The listing builds one solid part. Answer for the finished solid, in the listing's coordinates (mm). Face numbers are marked on the shaded views. Round coordinates to 2 decimals unless told otherwise and drop trailing zeros. Order: outer loops, then holes, each group sorted by start corner. A loop starts at its lowest first (then second) coordinate and runs counter-clockwise, first axis right, second up. Notation, with made-up numbers: (67.5, 60.5) -> (84.5, 60.5) arc R28 cw to (84.5, 79.5) -> close; hole circle Ø7 at (43.25, 60). An arc over 180 degrees is marked (long way). Answer in a Markdown table with one row per item. Add a question column.
```python
from build123d import *

# Parameters (mm, degrees)
F1_DEPTH = 1.2
F2_DEPTH = 10
F3_DEPTH = 7
F4_SIZE2 = 8
F4_SIZE  = 1.4


with BuildPart() as f1:
    # F0 (on Top) → F1 (new body)
    with BuildSketch(Plane.XY):
        with BuildLine():
            Line((81.8, 59.8), (-81.8, 59.8))
            ThreePointArc((-81.8, 59.8), (-83.9213203436, 58.9213203436), (-84.8, 56.8))
            Line((-84.8, 56.8), (-84.8, -56.8))
            ThreePointArc((-84.8, -56.8), (-83.9213203436, -58.9213203436), (-81.8, -59.8))
            Line((-81.8, -59.8), (81.8, -59.8))
            ThreePointArc((81.8, -59.8), (83.9213203436, -58.9213203436), (84.8, -56.8))
            Line((84.8, -56.8), (84.8, 56.8))
            ThreePointArc((84.8, 56.8), (83.9213203436, 58.9213203436), (81.8, 59.8))
        make_face()
        with BuildLine():
            ThreePointArc((83.2, -55.2), (82.3213203436, -57.3213203436), (80.2, -58.2))
            Line((80.2, -58.2), (-80.2, -58.2))
            ThreePointArc((-80.2, -58.2), (-82.3213203436, -57.3213203436), (-83.2, -55.2))
            Line((-83.2, -55.2), (-83.2, 55.2))
            ThreePointArc((-83.2, 55.2), (-82.3213203436, 57.3213203436), (-80.2, 58.2))
            Line((-80.2, 58.2), (80.2, 58.2))
            ThreePointArc((80.2, 58.2), (82.3213203436, 57.3213203436), (83.2, 55.2))
            Line((83.2, 55.2), (83.2, -55.2))
        make_face(mode=Mode.SUBTRACT)
        with BuildLine():
            Line((-80.2, -58.2), (80.2, -58.2))
            ThreePointArc((80.2, -58.2), (82.3213203436, -57.3213203436), (83.2, -55.2))
            Line((83.2, -55.2), (83.2, 55.2))
            ThreePointArc((83.2, 55.2), (82.3213203436, 57.3213203436), (80.2, 58.2))
            Line((80.2, 58.2), (-80.2, 58.2))
            ThreePointArc((-80.2, 58.2), (-82.3213203436, 57.3213203436), (-83.2, 55.2))
            Line((-83.2, 55.2), (-83.2, -55.2))
            ThreePointArc((-83.2, -55.2), (-82.3213203436, -57.3213203436), (-80.2, -58.2))
        make_face()
        with BuildLine():
            ThreePointArc((-81.2, 53.2), (-80.3213203436, 55.3213203436), (-78.2, 56.2))
            Line((-78.2, 56.2), (78.2, 56.2))
            ThreePointArc((78.2, 56.2), (80.3213203436, 55.3213203436), (81.2, 53.2))
            Line((81.2, 53.2), (81.2, -53.2))
            ThreePointArc((81.2, -53.2), (80.3213203436, -55.3213203436), (78.2, -56.2))
            Line((78.2, -56.2), (-78.2, -56.2))
            ThreePointArc((-78.2, -56.2), (-80.3213203436, -55.3213203436), (-81.2, -53.2))
            Line((-81.2, -53.2), (-81.2, 53.2))
        make_face(mode=Mode.SUBTRACT)
        with BuildLine():
            Line((78.2, 56.2), (-78.2, 56.2))
            ThreePointArc((-78.2, 56.2), (-80.3213203436, 55.3213203436), (-81.2, 53.2))
            Line((-81.2, 53.2), (-81.2, -53.2))
            ThreePointArc((-81.2, -53.2), (-80.3213203436, -55.3213203436), (-78.2, -56.2))
            Line((-78.2, -56.2), (78.2, -56.2))
            ThreePointArc((78.2, -56.2), (80.3213203436, -55.3213203436), (81.2, -53.2))
            Line((81.2, -53.2), (81.2, 53.2))
            ThreePointArc((81.2, 53.2), (80.3213203436, 55.3213203436), (78.2, 56.2))
        make_face()
        with BuildLine():
            ThreePointArc((-80, 52), (-79.1213203436, 54.1213203436), (-77, 55))
            Line((-77, 55), (77, 55))
            ThreePointArc((77, 55), (79.1213203436, 54.1213203436), (80, 52))
            Line((80, 52), (80, -52))
            ThreePointArc((80, -52), (79.1213203436, -54.1213203436), (77, -55))
            Line((77, -55), (-77, -55))
            ThreePointArc((-77, -55), (-79.1213203436, -54.1213203436), (-80, -52))
            Line((-80, -52), (-80, 52))
        make_face(mode=Mode.SUBTRACT)
        with BuildLine():
            Line((77, 55), (-77, 55))
            ThreePointArc((-77, 55), (-79.1213203436, 54.1213203436), (-80, 52))
            Line((-80, 52), (-80, -52))
            ThreePointArc((-80, -52), (-79.1213203436, -54.1213203436), (-77, -55))
            Line((-77, -55), (77, -55))
            ThreePointArc((77, -55), (79.1213203436, -54.1213203436), (80, -52))
            Line((80, -52), (80, 52))
            ThreePointArc((80, 52), (79.1213203436, 54.1213203436), (77, 55))
        make_face()
    extrude(amount=F1_DEPTH)

    # F0 (on Top) → F2 (join)
    with BuildSketch(Plane.XY):
        with BuildLine():
            Line((78.2, 56.2), (-78.2, 56.2))
            ThreePointArc((-78.2, 56.2), (-80.3213203436, 55.3213203436), (-81.2, 53.2))
            Line((-81.2, 53.2), (-81.2, -53.2))
            ThreePointArc((-81.2, -53.2), (-80.3213203436, -55.3213203436), (-78.2, -56.2))
            Line((-78.2, -56.2), (78.2, -56.2))
            ThreePointArc((78.2, -56.2), (80.3213203436, -55.3213203436), (81.2, -53.2))
            Line((81.2, -53.2), (81.2, 53.2))
            ThreePointArc((81.2, 53.2), (80.3213203436, 55.3213203436), (78.2, 56.2))
        make_face()
        with BuildLine():
            ThreePointArc((-80, 52), (-79.1213203436, 54.1213203436), (-77, 55))
            Line((-77, 55), (77, 55))
            ThreePointArc((77, 55), (79.1213203436, 54.1213203436), (80, 52))
            Line((80, 52), (80, -52))
            ThreePointArc((80, -52), (79.1213203436, -54.1213203436), (77, -55))
            Line((77, -55), (-77, -55))
            ThreePointArc((-77, -55), (-79.1213203436, -54.1213203436), (-80, -52))
            Line((-80, -52), (-80, 52))
        make_face(mode=Mode.SUBTRACT)
    extrude(amount=F2_DEPTH)

    # F0 (on Top) → F3 (join)
    with BuildSketch(Plane.XY):
        with BuildLine():
            Line((81.8, 59.8), (-81.8, 59.8))
            ThreePointArc((-81.8, 59.8), (-83.9213203436, 58.9213203436), (-84.8, 56.8))
            Line((-84.8, 56.8), (-84.8, -56.8))
            ThreePointArc((-84.8, -56.8), (-83.9213203436, -58.9213203436), (-81.8, -59.8))
            Line((-81.8, -59.8), (81.8, -59.8))
            ThreePointArc((81.8, -59.8), (83.9213203436, -58.9213203436), (84.8, -56.8))
            Line((84.8, -56.8), (84.8, 56.8))
            ThreePointArc((84.8, 56.8), (83.9213203436, 58.9213203436), (81.8, 59.8))
        make_face()
        with BuildLine():
            ThreePointArc((83.2, -55.2), (82.3213203436, -57.3213203436), (80.2, -58.2))
            Line((80.2, -58.2), (-80.2, -58.2))
            ThreePointArc((-80.2, -58.2), (-82.3213203436, -57.3213203436), (-83.2, -55.2))
            Line((-83.2, -55.2), (-83.2, 55.2))
            ThreePointArc((-83.2, 55.2), (-82.3213203436, 57.3213203436), (-80.2, 58.2))
            Line((-80.2, 58.2), (80.2, 58.2))
            ThreePointArc((80.2, 58.2), (82.3213203436, 57.3213203436), (83.2, 55.2))
            Line((83.2, 55.2), (83.2, -55.2))
        make_face(mode=Mode.SUBTRACT)
    extrude(amount=F3_DEPTH)

    # F4
    f4_edges = [f1.edges().sort_by_distance(p)[0] for p in [
        (-81.2, 0, 1.2),
    ]]
    chamfer(f4_edges, length=F4_SIZE, length2=F4_SIZE2)


solid = f1.part
```
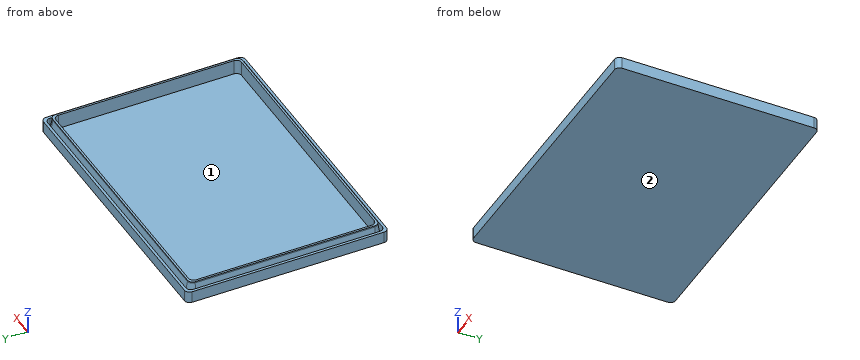
Item 1: The part is cut by section A-A, the plane z = 4. State how many separate pieces and enclosed holes the cut face has, and give its area (3 significant figures).
Item 2: The part is cut by section B-B, the plane y = 37.5. Give the vertices of the cut face in (x, z).
Item 3: The part is cut by section C-C, the plane x = -56. Give the vertices of the cut face in (y, z).
Item 4: Find the intervals of material crossed by probe 1 along X at (y, z) = (3.5, 5.75); probe 2 along X at (y, z) = (26.5, 9) (3 decimals); probe 3 along X at (y, z) = (39, 1.5), in increasing order. Write a range as [from, to].
Item 5: For a pull along X with two mould halves and no side action, classify the marked faces 1 and 2 as released by +X, released by -X, zero draft, split by the parting line, or undercut.
Item 6: A flat-ended cylindrical pin translates along its axis: P1, Ø2, axis at x = 5.5, z = 9, coming from the +Y side. Find the tip coordinate at first contact, or state that the pin passes through.
Resolved:
| question | item | result |
|---|---|---|
| 1 | separate pieces | 2 |
| 1 | enclosed holes | 2 |
| 1 | area | 2,070 mm2 |
| 2 | outline | (-84.8, 0) -> (84.8, 0) -> (84.8, 7) -> (83.2, 7) -> (83.2, 1.2) -> (82.6, 1.2) -> (81.2, 9.2) -> (81.2, 10) -> (80, 10) -> (80, 1.2) -> (-80, 1.2) -> (-80, 10) -> (-81.2, 10) -> (-81.2, 9.2) -> (-82.6, 1.2) -> (-83.2, 1.2) -> (-83.2, 7) -> (-84.8, 7) -> close |
| 3 | outline | (-59.8, 0) -> (59.8, 0) -> (59.8, 7) -> (58.2, 7) -> (58.2, 1.2) -> (57.6, 1.2) -> (56.2, 9.2) -> (56.2, 10) -> (55, 10) -> (55, 1.2) -> (-55, 1.2) -> (-55, 10) -> (-56.2, 10) -> (-56.2, 9.2) -> (-57.6, 1.2) -> (-58.2, 1.2) -> (-58.2, 7) -> (-59.8, 7) -> close |
| 4 | probe 1 | [-84.8, -83.2], [-81.8, -80], [80, 81.8], [83.2, 84.8] |
| 4 | probe 2 | [-81.235, -80], [80, 81.235] |
| 4 | probe 3 | [-84.8, -83.2], [-82.55, -80], [80, 82.55], [83.2, 84.8] |
| 5 | face 1 | undercut |
| 5 | face 2 | zero draft |
| 6 | P1 | y = 56.41 |
